Read the model definition and answer for the solid it produces. Units are mm, in the model's axes. Coordinates: 2 decimals unless noted, no trailing zeros. Write each loop counter-clockwise with the first axis right and the second up, starting at its lowest first coordinate (ties: lowest second). Pieces come first, ordered by that corner, then holes.
(1) Straight lines are drawn through the part: line 1 along Y through (x, z) = (0, -0.5) (3 decimals); line 2 along Y through (x, z) = (10, 0.55) (1 decimal); line 3 along Y through (x, z) = (-34, 0.65) (3 decimals). For each, find the intervals that lie inside material, in ascending order.
(2) The part is cut by section B-B, the plane x = 0. Determine the outline of the cut face in (y, z) (1 decimal).
(3) Determine the mould class of faces 1 (the flat face through (57.187, -65.501, -0.022)), 2 (the cylindrical face through (-23.651, -76.475, -0.022)) for opening direction Y: pulls with the +Y half, pulls with the -Y half, needs draft (parallel to the pull), parting line crosses it, or undercut.
(4) The part is cut by section A-A, the plane y = -50.8. State how many separate pieces and enclosed holes the cut face has, and give its area (3 significant figures).
```python
from build123d import *

# Parameters (mm, degrees)
SKETCH1_W           = 199.39
SKETCH1_H           = 69.85
SKETCH1_R           = 12.7
SKETCH1_W_2         = 6.35
SKETCH1_H_2         = 44.45
BOSS_EXTRUDE1_DEPTH = 1.5875
SKETCH1_3_W         = 6.35
SKETCH1_3_H         = 44.45
CUT_EXTRUDE1_DEPTH  = 3.175
FILLET1_R           = 2.54


with BuildPart() as part:
    # Sketch1 → Boss-Extrude1 (new body, symmetric)
    with BuildSketch(Plane.XY):
        with Locations((0, -50.8)):
            Rectangle(SKETCH1_W, SKETCH1_H)
        with Locations((0, -50.8)):
            Circle(SKETCH1_R, mode=Mode.SUBTRACT)
        with Locations((88.9, -50.8)):
            Rectangle(SKETCH1_W_2, SKETCH1_H_2, mode=Mode.SUBTRACT)
    extrude(amount=BOSS_EXTRUDE1_DEPTH, both=True)

    # Sketch1_3 → Cut-Extrude1 (cut, symmetric)
    with BuildSketch(Plane.XY):
        with BuildLine():
            Line((39.696193404, -50.8), (23.976512651, -37.587857063))
            ThreePointArc((23.976512651, -37.587857063), (27.375790032, -50.8), (23.976512651, -64.012142937))
            Line((23.976512651, -64.012142937), (39.696193404, -50.8))
        make_face()
        Polygon((72.183420116, -23.495), (19.052126459, -23.495), (45.617773288, -45.823005806), align=None)
        Polygon((78.105, -28.471994194), (51.539353171, -50.8), (78.105, -73.128005806), align=None)
        Polygon((72.183420116, -78.105), (45.617773288, -55.776994194), (19.052126459, -78.105), align=None)
        with Locations((88.9, -50.8)):
            Rectangle(SKETCH1_3_W, SKETCH1_3_H)
        with BuildLine():
            Line((23.976512651, -37.587857063), (8.89, -24.907881896))
            Line((8.89, -24.907881896), (8.89, -32.527881896))
            ThreePointArc((8.89, -32.527881896), (20.32, -50.8), (8.89, -69.072118104))
            Line((8.89, -69.072118104), (8.89, -76.692118104))
            Line((8.89, -76.692118104), (23.976512651, -64.012142937))
            ThreePointArc((23.976512651, -64.012142937), (27.375790032, -50.8), (23.976512651, -37.587857063))
        make_face()
    cut_extrude1 = extrude(amount=CUT_EXTRUDE1_DEPTH, both=True, mode=Mode.SUBTRACT)

    # Mirror1: Cut-Extrude1 across plane
    add(cut_extrude1.mirror(Plane(origin=(0, 0, 0), x_dir=(0, 0, 1), z_dir=(1, 0, 0))), mode=Mode.SUBTRACT)

    # Fillet1
    fillet1_edges = [part.edges().sort_by_distance(p)[0] for p in [
        (-72.183420116, -78.105, 0),
        (-45.617773288, -55.776994194, 0),
        (-19.052126459, -78.105, 0),
        (-78.105, -73.128005806, 0),
        (-78.105, -28.471994194, 0),
        (-51.539353171, -50.8, 0),
        (-39.696193404, -50.8, 0),
        (-8.89, -24.907881896, 0),
        (-8.89, -32.527881896, 0),
        (-8.89, -69.072118104, 0),
        (-8.89, -76.692118104, 0),
        (99.695, -85.725, 0),
        (-99.695, -85.725, 0),
        (-99.695, -15.875, 0),
        (99.695, -15.875, 0),
        (-19.052126459, -23.495, 0),
        (-45.617773288, -45.823005806, 0),
        (-72.183420116, -23.495, 0),
        (45.617773288, -55.776994194, 0),
        (72.183420116, -78.105, 0),
        (19.052126459, -78.105, 0),
        (78.105, -28.471994194, 0),
        (78.105, -73.128005806, 0),
        (51.539353171, -50.8, 0),
        (8.89, -24.907881896, 0),
        (39.696193404, -50.8, 0),
        (8.89, -76.692118104, 0),
        (8.89, -69.072118104, 0),
        (8.89, -32.527881896, 0),
        (45.617773288, -45.823005806, 0),
        (19.052126459, -23.495, 0),
        (72.183420116, -23.495, 0),
    ]]
    fillet(fillet1_edges, radius=FILLET1_R)


solid = part.part
```
Computed:
1. line 1: y = -85.725 to -63.5, -38.1 to -15.875
1. line 2: y = -85.7 to -73.3, -68.5 to -58.6, -43 to -33.1, -28.3 to -15.9
1. line 3: y = -85.725 to -78.105, -65.542 to -55.588, -46.012 to -36.058, -23.495 to -15.875
2. outline: (-85.7, -1.6) - (-63.5, -1.6) - (-63.5, 1.6) - (-85.7, 1.6) - close; (-38.1, -1.6) - (-15.9, -1.6) - (-15.9, 1.6) - (-38.1, 1.6) - close
3. face 1: undercut
3. face 2: undercut
4. separate pieces: 8
4. enclosed holes: 0
4. area: 238 mm2
